Build history of the part. All positions in model axes, mm. A direction names the side the tool comes from. Give positions to 0.01 mm unless a question says otherwise; leave off trailing zeros. Write each loop counter-clockwise with the first axis right and the second up, starting at its lowest first coordinate (ties: lowest second). Pieces come first, ordered by that corner, then holes.
from build123d import *

# Parameters (mm, degrees)
SKETCH1_R           = 1.625
BOSS_EXTRUDE1_DEPTH = 5
BOSS_EXTRUDE2_START = 5
SKETCH1_3_W         = 20
SKETCH1_3_H         = 70
BOSS_EXTRUDE2_DEPTH = 10.5
BOSS_EXTRUDE3_START = 15.5
SKETCH1_4_R         = 1.625
BOSS_EXTRUDE3_DEPTH = 5
SKETCH1_5_W         = 9
SKETCH1_5_H         = 12
SKETCH1_5_W_2       = 11
BOSS_EXTRUDE4_DEPTH = 5
BOSS_EXTRUDE5_START = 15.5
SKETCH1_6_W         = 9
SKETCH1_6_H         = 12
SKETCH1_6_W_2       = 11
BOSS_EXTRUDE5_DEPTH = 5
SKETCH2_R           = 1.5
BOSS_EXTRUDE6_DEPTH = 10
CUT_EXTRUDE1_START  = 10
SKETCH2_3_R         = 1.5
CUT_EXTRUDE1_DEPTH  = 10
CUT_EXTRUDE2_START  = -120
SKETCH3_R           = 3.81
CUT_EXTRUDE2_DEPTH  = 20


with BuildPart() as part:
    # Sketch1 → Boss-Extrude1 (new body)
    with BuildSketch(Plane.XY):
        Polygon((20, 70), (29, 70), (29, 80), (49, 80), (49, 70), (60, 70), (60, 95), (0, 95), (0, 0), (20, 0), align=None)
        with Locations((34.9, 90.3)):
            Circle(SKETCH1_R, mode=Mode.SUBTRACT)
        with Locations((57.1, 80)):
            Circle(SKETCH1_R, mode=Mode.SUBTRACT)
    extrude(amount=BOSS_EXTRUDE1_DEPTH)

    # Sketch1<3> → Boss-Extrude2 (add)
    with BuildSketch(Plane.XY.offset(BOSS_EXTRUDE2_START)):
        with Locations((10, 35)):
            Rectangle(SKETCH1_3_W, SKETCH1_3_H)
    extrude(amount=BOSS_EXTRUDE2_DEPTH)

    # Sketch1<4> → Boss-Extrude3 (add)
    with BuildSketch(Plane.XY.offset(BOSS_EXTRUDE3_START)):
        Polygon((20, 70), (29, 70), (29, 80), (49, 80), (49, 70), (60, 70), (60, 95), (0, 95), (0, 0), (20, 0), align=None)
        with Locations((34.9, 90.3)):
            Circle(SKETCH1_4_R, mode=Mode.SUBTRACT)
        with Locations((57.1, 80)):
            Circle(SKETCH1_4_R, mode=Mode.SUBTRACT)
    extrude(amount=BOSS_EXTRUDE3_DEPTH)

    # Sketch1<5> → Boss-Extrude4 (add)
    with BuildSketch(Plane.XY):
        with Locations((24.5, 64)):
            Rectangle(SKETCH1_5_W, SKETCH1_5_H)
        with Locations((54.5, 64)):
            Rectangle(SKETCH1_5_W_2, SKETCH1_5_H)
    extrude(amount=BOSS_EXTRUDE4_DEPTH)

    # Sketch1<6> → Boss-Extrude5 (add)
    with BuildSketch(Plane.XY.offset(BOSS_EXTRUDE5_START)):
        with Locations((24.5, 64)):
            Rectangle(SKETCH1_6_W, SKETCH1_6_H)
        with Locations((54.5, 64)):
            Rectangle(SKETCH1_6_W_2, SKETCH1_6_H)
    extrude(amount=BOSS_EXTRUDE5_DEPTH)

    # Sketch2 → Boss-Extrude6 (add)
    with BuildSketch(Plane(origin=(0, 0, 0), x_dir=(0, 0, -1), z_dir=(1, 0, 0))):
        Polygon((4.75, 65), (4.75, 95), (-5, 95), (-5, 70), (-15.5, 70), (-15.5, 95), (-25.25, 95), (-25.25, 65), align=None)
        with Locations((-20.25, 71)):
            Circle(SKETCH2_R, mode=Mode.SUBTRACT)
        with Locations((-0.25, 71)):
            Circle(SKETCH2_R, mode=Mode.SUBTRACT)
        with Locations((-20.25, 91)):
            Circle(SKETCH2_R, mode=Mode.SUBTRACT)
        with Locations((-0.25, 91)):
            Circle(SKETCH2_R, mode=Mode.SUBTRACT)
    extrude(amount=-BOSS_EXTRUDE6_DEPTH)

    # Sketch2<3> → Cut-Extrude1 (cut)
    with BuildSketch(Plane(origin=(0, 0, 0), x_dir=(0, 0, -1), z_dir=(1, 0, 0)).offset(CUT_EXTRUDE1_START)):
        with Locations((-0.25, 91)):
            Circle(SKETCH2_3_R)
        with Locations((-20.25, 91)):
            Circle(SKETCH2_3_R)
        with Locations((-20.25, 71)):
            Circle(SKETCH2_3_R)
        with Locations((-0.25, 71)):
            Circle(SKETCH2_3_R)
    extrude(amount=-CUT_EXTRUDE1_DEPTH, mode=Mode.SUBTRACT)

    # Sketch3 → Cut-Extrude2 (cut)
    with BuildSketch(Plane.ZY.offset(100).offset(CUT_EXTRUDE2_START)):
        with Locations(Location((10.25, 21, 0), (0, 0, 90))):
            Circle(SKETCH3_R)
    extrude(amount=CUT_EXTRUDE2_DEPTH, mode=Mode.SUBTRACT)


solid = part.part
1. Saw through at D-D on x = 34.9. Give the cut face in (y, z) (3 decimals), plus the area to 4 significant figures.
2. Saw through at B-B on y = 66. Give the cut face in (x, z), plus the area to 3 significant figures.
3. Drop flat-ended pins along their axis: pin 1 (5 mm diameter, centred on x = 57.1, y = 80, fed in from -Z); pin 2 (10 mm diameter, centred on x = 32, z = 0, fed in from -Y); pin 3 (1 mm diameter, centred on x = 17, z = 12, fed in from +Y); pin 4 (5 mm diameter, centred on x = 8, z = 14, fed in from +Y). Give the stop position or say it passes through.
4. Mould opens along Z. For faces 1 (the face through (23, 59, 20.5)), 2 (the face through (10.14, 24.634, 9.106)), 3 (the face through (60, 76, 18)) say: pulls with the +Z half, pulls with the -Z half, needs draft (parallel to the pull), parting line crosses it, or undercut.
5. Drill centre lines: line 1 along Z through (x, y) = (-2, 71); line 2 along Z through (x, y) = (27, 63); line 3 along X through (y, z) = (90.3, 17.15) (3 decimals). Where is each one in solid material? Low to high.
6. Saw through at C-C on y = 21. Give the cut face in (x, z).
7. Saw through at A-A on x = 46. Give the cut face in (y, z), plus the area to 3 significant figures.
8. 3-axis set-ups, long thin cutter, end or side, ignore diameter. For faces 4 (the face through (29, 69, 18)), 5 (the face through (-5, 65, 10)), 6 (the face through (-2.08, 71.07, 1.75)), 7 (the face through (24, 58, 2)): which of +Z, -Z, +X, -X, +Y, -Y reach the whole face in a straight line?
Outcome:
1. outline: (80, 0) - (88.675, 0) - (88.675, 5) - (80, 5) - close; (80, 15.5) - (88.675, 15.5) - (88.675, 20.5) - (80, 20.5) - close; (91.925, 0) - (95, 0) - (95, 5) - (91.925, 5) - close; (91.925, 15.5) - (95, 15.5) - (95, 20.5) - (91.925, 20.5) - close
1. area: 117.5 mm2
2. outline: (-10, -4.75) - (0, -4.75) - (0, 0) - (29, 0) - (29, 5) - (20, 5) - (20, 15.5) - (29, 15.5) - (29, 20.5) - (0, 20.5) - (0, 25.25) - (-10, 25.25) - close; (49, 0) - (60, 0) - (60, 5) - (49, 5) - close; (49, 15.5) - (60, 15.5) - (60, 20.5) - (49, 20.5) - close
2. area: 910 mm2
3. pin 1: stops at z = 0
3. pin 2: stops at y = 58
3. pin 3: stops at y = 70
3. pin 4: stops at y = 95
4. face 1: pulls with the +Z half
4. face 2: undercut
4. face 3: needs draft
5. line 1: z = -4.75 to -1.25, 1.75 to 5, 15.5 to 18.75, 21.75 to 25.25
5. line 2: z = 0 to 5, 15.5 to 20.5
5. line 3: x = -10 to 33.275, 36.525 to 60
6. outline: (0, 0) - (20, 0) - (20, 6.44) - (0, 6.44) - close; (0, 14.06) - (20, 14.06) - (20, 20.5) - (0, 20.5) - close
7. outline: (80, 0) - (95, 0) - (95, 5) - (80, 5) - close; (80, 15.5) - (95, 15.5) - (95, 20.5) - (80, 20.5) - close
7. area: 150 mm2
8. face 4: +Z, -Z, -Y
8. face 5: +Z, -Z, -X, -Y
8. face 6: -X
8. face 7: +Z, -Z, +X, -Y
